Verification items for the finished model (mm, model axes). Face numbers are marked on the shaded views. A direction names the side the tool comes from. Round coordinates to 2 decimals unless told otherwise and drop trailing zeros. Loops run counter-clockwise (first coordinate to the right, second up) from the corner with the lowest first, then second, coordinate; pieces in that order, holes last. Notation, with made-up numbers: M -10.5,-20 L 17.5,-20 A19 cw 17.5,-4 Z; hole C 61.5,21 d6. An arc over 180 degrees is marked long. Answer as CSV lines item,"result".
```python
from build123d import *

# Parameters (mm, degrees)
SKETCH2_R           = 11
BOSS_EXTRUDE1_DEPTH = 20
SKETCH3_R           = 10
BOSS_EXTRUDE2_DEPTH = 8
SKETCH4_W           = 8
SKETCH4_H           = 12
CUT_EXTRUDE1_DEPTH  = 3.7
SKETCH6_OUTSIDE_W   = 36.812
SKETCH6_OUTSIDE_H   = 36.812
SKETCH6_OUTSIDE_R   = 10
CUT_EXTRUDE4_DEPTH  = 1.75


with BuildPart() as part:
    # Sketch2 → Boss-Extrude1 (new body)
    with BuildSketch(Plane.XY):
        Circle(SKETCH2_R)
    extrude(amount=BOSS_EXTRUDE1_DEPTH)

    # Sketch3 → Boss-Extrude2 (add)
    with BuildSketch(Plane.XY.offset(20)):
        Circle(SKETCH3_R)
    extrude(amount=BOSS_EXTRUDE2_DEPTH)

    # Mirror1: part across plane


with BuildPart() as part_1:
    add(part.part)
    add(part.part.mirror(Plane.XY))

    # Sketch4 → Cut-Extrude1 (cut)
    with BuildSketch(Plane(origin=(0, 11, 0), x_dir=(1, 0, 0), z_dir=(0, 1, 0))):
        Rectangle(SKETCH4_W, SKETCH4_H)
        with BuildLine():
            ThreePointArc((-4, 6), (0, 10), (4, 6))
            Line((4, 6), (-4, 6))
        make_face()
        with BuildLine():
            Line((-4, -6), (4, -6))
            ThreePointArc((4, -6), (0, -10), (-4, -6))
        make_face()
    extrude(amount=-CUT_EXTRUDE1_DEPTH, mode=Mode.SUBTRACT)

    # Sketch6 outside → Cut-Extrude4 (cut)
    with BuildSketch(Plane.XY.offset(11)):
        Rectangle(SKETCH6_OUTSIDE_W, SKETCH6_OUTSIDE_H)
        Circle(SKETCH6_OUTSIDE_R, mode=Mode.SUBTRACT)
    cut_extrude4 = extrude(amount=CUT_EXTRUDE4_DEPTH, mode=Mode.SUBTRACT)

    # Mirror2: Cut-Extrude4 across plane
    add(cut_extrude4.mirror(Plane.XY), mode=Mode.SUBTRACT)


solid = part_1.part
```
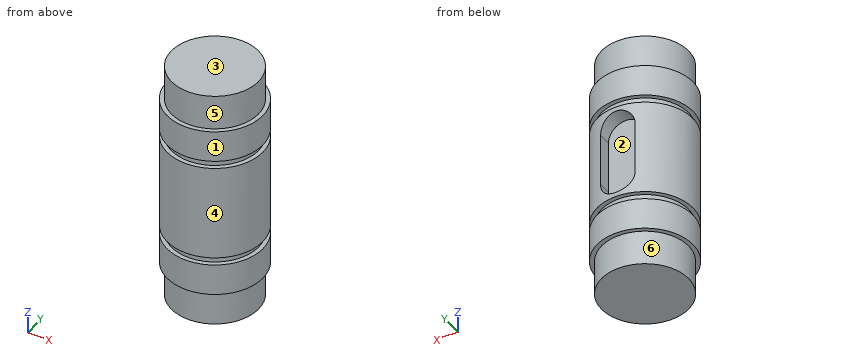
1) Go/stop test with flat-tipped pins: pin 1 (1.5 mm diameter, centred on x = 5, z = -9, fed in from -Y); pin 2 (8 mm diameter, centred on y = 5.5, z = -14.5, fed in from -X); pin 3 (2.5 mm diameter, centred on y = 9, z = 0.5, fed in from +X). Record where each tip stops, or that it passes through.
Here are the results:
pin 1,"stops at y = -10.15"
pin 2,"stops at x = -10.9"
pin 3,"stops at x = 7.81"
2) Draft check along X on the marked faces 1, 2 and 3. Enter one of: +X half, -X half, draft (parallel to the pull), parting line (faces both ways), or undercut.
Here are the results:
face 1,"parting line"
face 2,"undercut"
face 3,"draft"
3) Section check B-B (y = 0). Record the cut outline in (x, z).
Here are the results:
outline,"M -11,-20 L -10,-20 L -10,-28 L 10,-28 L 10,-20 L 11,-20 L 11,-12.75 L 10,-12.75 L 10,-11 L 11,-11 L 11,11 L 10,11 L 10,12.75 L 11,12.75 L 11,20 L 10,20 L 10,28 L -10,28 L -10,20 L -11,20 L -11,12.75 L -10,12.75 L -10,11 L -11,11 L -11,-11 L -10,-11 L -10,-12.75 L -11,-12.75 Z"
4) Material ranges on probe 1 along Z at (x, y) = (3.5, 9.25); probe 2 along Y at (x, z) = (4.75, 21.5); probe 3 along X at (y, z) = (6.5, 19.5), recorded low to high.
Here are the results:
probe 1,"z = -28 to -7.94, 7.94 to 28"
probe 2,"y = -8.8 to 8.8"
probe 3,"x = -8.87 to 8.87"
5) Section check D-D (z = 23). Record the cut outline in (x, y), plus the area to 3 significant figures.
Here are the results:
outline,"C 0,0 d20"
area,"314 mm^2"
6) Set-up check for the marked faces 4, 5 and 6: record each of +Z, -Z, +X, -X, +Y, -Y from which the full face is reachable in a straight line by a thin tool's end or side.
Here are the results:
face 4,"+Z, -Z"
face 5,"+Z"
face 6,"-Z"
